For this review, take the finished solid that the model builds, in its own axes (mm). A direction names the side the tool comes from. Give positions to 0.01 mm unless a question says otherwise; leave off trailing zeros. Order: outer loops, then holes, each group sorted by start corner. A loop starts at its lowest first (then second) coordinate and runs counter-clockwise, first axis right, second up. Notation, with made-up numbers: (36.25, -16) - (48.25, -16) arc R9 cw to (48.25, -1) - close; hole circle Ø5 at (21, -13). An arc over 180 degrees is marked (long way). One line per item, written item: value.
```python
from build123d import *

# Parameters (mm, degrees)
F0_R     = 6.35
F1_DEPTH = 6.35
F2_DEPTH = 7.62


with BuildPart() as f1:
    # F0 (on Top) → F1 (new body)
    with BuildSketch(Plane.XY):
        Polygon((-29.197408, 4.85902), (-41.897408, 4.85902), (-41.897408, -7.84098), (-41.897408, -33.24098), (-41.897408, -45.94098), (34.302592, -45.94098), (34.302592, 4.85902), (21.602592, 4.85902), (-3.797408, 4.85902), align=None)
        with Locations((-29.197408, -33.24098)):
            Circle(F0_R, mode=Mode.SUBTRACT)
        with Locations((-3.797408, -33.24098)):
            Circle(F0_R, mode=Mode.SUBTRACT)
        with Locations((21.602592, -33.24098)):
            Circle(F0_R, mode=Mode.SUBTRACT)
        with Locations((-29.197408, -7.84098)):
            Circle(F0_R, mode=Mode.SUBTRACT)
        with Locations((-3.797408, -7.84098)):
            Circle(F0_R, mode=Mode.SUBTRACT)
        with Locations((21.602592, -7.84098)):
            Circle(F0_R, mode=Mode.SUBTRACT)
    extrude(amount=F1_DEPTH)

    # F0 (on Top) → F2 (join)
    with BuildSketch(Plane.XY):
        with Locations((21.602592, -7.84098)):
            Circle(F0_R)
        with Locations((-3.797408, -7.84098)):
            Circle(F0_R)
        with Locations((-29.197408, -7.84098)):
            Circle(F0_R)
        with Locations((-29.197408, -33.24098)):
            Circle(F0_R)
        with Locations((-3.797408, -33.24098)):
            Circle(F0_R)
        with Locations((21.602592, -33.24098)):
            Circle(F0_R)
    extrude(amount=F2_DEPTH)


solid = f1.part
```
(1) For P1, Ø1, axis at x = -32.5, y = -0.5, coming from the +Z side, flat-tipped, find the tip position at first contact; note if it passes through.
Answers below:
P1: stops at z = 6.35
(2) Draft analysis for pull direction X (two halves, no side actions). For faces 3 (the face through (34.303, -21, 3)), 4 (the face through (27.66, -5.93, 6.98)), 5 (the face through (-4, -20, 0)), state which applies: pulls with the +X half, pulls with the -X half, needs draft (parallel to the pull), parting line crosses it, or undercut.
Answers below:
face 3: pulls with the +X half
face 4: undercut
face 5: needs draft
(3) Wall thickness on line 1 (X direction, y = -3, z = 6.75); line 2 (X direction, y = -31, z = 7.25); line 3 (Z direction, x = 31, y = -17): over which ranges is each line inside the solid? List them lowest first. Write a range as from..to.
Answers below:
line 1: x = -33.31..-25.09, -7.91..0.31, 17.49..25.71
line 2: x = -35.14..-23.26, -9.74..2.14, 15.66..27.54
line 3: z = 0..6.35
(4) Take a section at D-D (x = -25). Write out the cut boundary in (y, z), then the cut area to 3 significant figures.
Answers below:
outline: (-45.94, 0) - (4.86, 0) - (4.86, 6.35) - (-3.08, 6.35) - (-3.08, 7.62) - (-12.61, 7.62) - (-12.61, 6.35) - (-28.48, 6.35) - (-28.48, 7.62) - (-38.01, 7.62) - (-38.01, 6.35) - (-45.94, 6.35) - close
area: 347 mm^2
(5) Machinability: for faces 1 (the face through (22, -8, 7.62)), 2 (the face through (-23.33, -35.67, 6.98)), which of the approach directions +Z, -Z, +X, -X, +Y, -Y give a long, thin tool a straight path to every point of the face, cutting with its end or side? Answer none if there is none.
Answers below:
face 1: +Z, +X, -X, +Y, -Y
face 2: +Z
(6) Take a section at A-A (x = 1). Write out the cut boundary in (y, z), then the cut area to 3 significant figures.
Answers below:
outline: (-45.94, 0) - (4.86, 0) - (4.86, 6.35) - (-3.68, 6.35) - (-3.68, 7.62) - (-12, 7.62) - (-12, 6.35) - (-29.08, 6.35) - (-29.08, 7.62) - (-37.4, 7.62) - (-37.4, 6.35) - (-45.94, 6.35) - close
area: 344 mm^2
(7) Take a section at B-B (y = -5). Write out the cut boundary in (x, z), then the cut area to 3 significant figures.
Answers below:
outline: (-41.9, 0) - (34.3, 0) - (34.3, 6.35) - (27.28, 6.35) - (27.28, 7.62) - (15.92, 7.62) - (15.92, 6.35) - (1.88, 6.35) - (1.88, 7.62) - (-9.48, 7.62) - (-9.48, 6.35) - (-23.52, 6.35) - (-23.52, 7.62) - (-34.88, 7.62) - (-34.88, 6.35) - (-41.9, 6.35) - close
area: 527 mm^2
(8) Take a section at C-C (y = -34.5). Write out the cut boundary in (x, z).
Answers below:
outline: (-41.9, 0) - (34.3, 0) - (34.3, 6.35) - (27.83, 6.35) - (27.83, 7.62) - (15.38, 7.62) - (15.38, 6.35) - (2.43, 6.35) - (2.43, 7.62) - (-10.02, 7.62) - (-10.02, 6.35) - (-22.97, 6.35) - (-22.97, 7.62) - (-35.42, 7.62) - (-35.42, 6.35) - (-41.9, 6.35) - close
